The model under review builds one solid part; all positions refer to its coordinate system, in mm. A direction names the side the tool comes from. Coordinates: 2 decimals unless noted, no trailing zeros. Write each loop counter-clockwise with the first axis right and the second up, starting at its lowest first coordinate (ties: lowest second). Pieces come first, ordered by that corner, then holes.
1) Add section B-B, the plane z = -34.5. State the section outline as (x, y) points.
2) Mouldability with a two-part tool opening along Z and no side actions: class faces 4 (the flat face through (0, 2, -30)), 5 (the flat face through (18.75, 2, -20)), 6 (the flat face through (9.137, 2, -21)) as released by +Z, released by -Z, zero draft, split by the parting line, or undercut.
3) Machinability: for faces 1 (the flat face through (0, 2, 0)), 2 (the flat face through (10, 2, -35.5)), 3 (the flat face through (1.65, 2, -35)), which of the approach directions +Z, -Z, +X, -X, +Y, -Y give a long, thin tool a straight path to every point of the face, cutting with its end or side? Answer none if there is none.
4) For line 1 (X direction, y = 0.7, z = -14); line 2 (X direction, y = 1.4, z = -32); line 3 (Z direction, x = 12.5, y = 1.95), list the stretches that pass through material, from the lowest coordinate up.
5) Add section C-C, the plane z = -22. State the section outline as (x, y) points, then the cut area to 3 significant figures.
6) Add section D-D, the plane y = 1.5. Give the number of separate pieces and of enclosed holes in the cut face, then the cut area to 3 significant figures.
7) For P1, Ø3, axis at x = 3, z = -35.5, coming from the -Y side, flat-tipped, find the tip position at first contact; note if it passes through.
8) Add section A-A, the plane z = -2.5. State the section outline as (x, y) points.
from build123d import *

# Parameters (mm, degrees)
BOSS_EXTRUDE1_DEPTH                = 3.05
FILLET3_R                          = 0.5
SKETCH2_W                          = 3.3
SKETCH2_H                          = 46
SKETCH2_H_2                        = 1
CUT_EXTRUDE1_DEPTH                 = 45.945689448
SKETCH6_W                          = 2
SKETCH6_H                          = 23
CUT_EXTRUDE2_DEPTH                 = 45.945689448
FILLET4_R                          = 0.5
M3_CLEARANCE_HEAD_MOUNTING_HOLES_D = 3.2
SKETCH7_W                          = 0.5
SKETCH7_H                          = 40.5
CUT_EXTRUDE3_DEPTH                 = 45.945689448


with BuildPart() as part:
    # Sketch1 → Boss-Extrude1 (new body)
    with BuildSketch(Plane(origin=(0, 0, 0), x_dir=(1, 0, 0), z_dir=(0, 1, 0))):
        Polygon((-19.25, 0), (-19.25, 40.5), (-12.25, 40.5), (-15.136751346, 35.5), (-5.136751346, 35.5), (-8.023502692, 40.5), (8.023502692, 40.5), (5.136751346, 35.5), (15.136751346, 35.5), (12.25, 40.5), (19.25, 40.5), (19.25, 0), align=None)
    extrude(amount=BOSS_EXTRUDE1_DEPTH)

    # Fillet3
    fillet3_edges = [part.edges().sort_by_distance(p)[0] for p in [
        (-12.25, 1.525, -40.5),
        (-15.136751346, 1.525, -35.5),
        (-5.136751346, 1.525, -35.5),
        (-8.023502692, 1.525, -40.5),
        (8.023502692, 1.525, -40.5),
        (5.136751346, 1.525, -35.5),
        (15.136751346, 1.525, -35.5),
        (12.25, 1.525, -40.5),
    ]]
    fillet(fillet3_edges, radius=FILLET3_R)

    # Sketch2 → Cut-Extrude1 (cut, through all)
    with BuildSketch(Plane(origin=(0, 3.05, 0), x_dir=(1, 0, 0), z_dir=(0, 1, 0))):
        with Locations((0, 53)):
            Rectangle(SKETCH2_W, SKETCH2_H)
        with Locations((0, 28.3)):
            Rectangle(SKETCH2_W, SKETCH2_H_2)
    extrude(amount=-CUT_EXTRUDE1_DEPTH, mode=Mode.SUBTRACT)

    # Sketch6 → Cut-Extrude2 (cut, through all)
    with BuildSketch(Plane(origin=(0, 3.05, 0), x_dir=(1, 0, 0), z_dir=(0, 1, 0))):
        with Locations((-10.136751346, 21)):
            Rectangle(SKETCH6_W, SKETCH6_H)
        with Locations((10.136751346, 21)):
            Rectangle(SKETCH6_W, SKETCH6_H)
    extrude(amount=-CUT_EXTRUDE2_DEPTH, mode=Mode.SUBTRACT)

    # Fillet4
    fillet4_edges = [part.edges().sort_by_distance(p)[0] for p in [
        (-11.136751346, 1.525, -9.5),
        (-11.136751346, 1.525, -32.5),
        (-9.136751346, 1.525, -32.5),
        (-9.136751346, 1.525, -9.5),
        (11.136751346, 1.525, -32.5),
        (11.136751346, 1.525, -9.5),
        (9.136751346, 1.525, -9.5),
        (9.136751346, 1.525, -32.5),
    ]]
    fillet(fillet4_edges, radius=FILLET4_R)

    # M3 Clearance Head Mounting Holes (through all)
    with Locations(Plane(origin=(0, 3.05, 0), x_dir=(1, 0, 0), z_dir=(0, 1, 0))):
        with Locations((-12.5, 2.5), (12.5, 2.5)):
            Hole(M3_CLEARANCE_HEAD_MOUNTING_HOLES_D / 2)

    # Sketch7 → Cut-Extrude3 (cut, through all)
    with BuildSketch(Plane(origin=(0, 3.05, 0), x_dir=(1, 0, 0), z_dir=(0, 1, 0))):
        with Locations((-19, 20.25)):
            Rectangle(SKETCH7_W, SKETCH7_H)
        with Locations((19, 20.25)):
            Rectangle(SKETCH7_W, SKETCH7_H)
    extrude(amount=-CUT_EXTRUDE3_DEPTH, mode=Mode.SUBTRACT)


solid = part.part
Geometry results:
1. outline: (-18.75, 0) - (-1.65, 0) - (-1.65, 3.05) - (-18.75, 3.05) - close; (1.65, 0) - (18.75, 0) - (18.75, 3.05) - (1.65, 3.05) - close
2. face 4: released by -Z
2. face 5: zero draft
2. face 6: undercut
3. face 1: +Z, +X, -X, +Y, -Y
3. face 2: +Y, -Y
3. face 3: -Z, +Y, -Y
4. line 1: x = -18.75 to -11.14, -9.14 to 9.14, 11.14 to 18.75
4. line 2: x = -18.75 to -11.14, -9.14 to -1.65, 1.65 to 9.14, 11.14 to 18.75
4. line 3: z = -35.5 to -4.1, -0.9 to 0
5. outline: (-18.75, 0) - (-11.14, 0) - (-11.14, 3.05) - (-18.75, 3.05) - close; (-9.14, 0) - (9.14, 0) - (9.14, 3.05) - (-9.14, 3.05) - close; (11.14, 0) - (18.75, 0) - (18.75, 3.05) - (11.14, 3.05) - close
5. area: 102 mm2
6. separate pieces: 1
6. enclosed holes: 5
6. area: 1,300 mm2
7. P1: stops at y = 0
8. outline: (-18.75, 0) - (-14.1, 0) - (-14.1, 3.05) - (-18.75, 3.05) - close; (-10.9, 0) - (10.9, 0) - (10.9, 3.05) - (-10.9, 3.05) - close; (14.1, 0) - (18.75, 0) - (18.75, 3.05) - (14.1, 3.05) - close
